Could you check a few things on this model? Use its own coordinates, in mm. Coordinates: 2 decimals unless noted, no trailing zeros. Write each loop counter-clockwise with the first axis right and the second up, starting at its lowest first coordinate (ties: lowest second). Pieces come first, ordered by that corner, then holes. Notation, with made-up numbers: M 54,48.5 L 92,48.5 A10 ccw 92,63.5 Z; hole C -14,46 d6. An arc over 180 degrees is marked long. Write item = value, one per line.
```python
from build123d import *

# Parameters (mm, degrees)
BOSS_EXTRUDE1_DEPTH = 6
SKETCH2_R           = 2.25
CUT_EXTRUDE1_DEPTH  = 20


with BuildPart() as part:
    # Sketch1 → Boss-Extrude1 (new, symmetric)
    with BuildSketch(Plane(origin=(0, 0, 0), x_dir=(0, 0, -1), z_dir=(1, 0, 0))):
        with BuildLine():
            Line((-1, 7.433034374), (-1, 15))
            Line((-1, 15), (-11, 15))
            Line((-11, 15), (-11, -15))
            Line((-11, -15), (-1, -15))
            Line((-1, -15), (-1, -7.433034374))
            ThreePointArc((-1, -7.433034374), (-7.5, 0), (-1, 7.433034374))
        make_face()
    extrude(amount=BOSS_EXTRUDE1_DEPTH, both=True)

    # Sketch2 → Cut-Extrude1 (cut, through all)
    with BuildSketch(Plane.XY.offset(11)):
        with Locations((0, 11)):
            Circle(SKETCH2_R)
        with Locations((0, -11)):
            Circle(SKETCH2_R)
    extrude(amount=-CUT_EXTRUDE1_DEPTH, mode=Mode.SUBTRACT)


solid = part.part
```
Item 1: Imagine slicing it at A-A (y = -11). Write out the boundary of the cut face in (x, z).
Numbers:
outline = M -6,1 L -2.25,1 L -2.25,11 L -6,11 Z; M 2.25,1 L 6,1 L 6,11 L 2.25,11 Z
Item 2: If we mould it in two halves opening along Y, with no side actions, what happens to faces 1 (the face through (-0.29, -8.77, 6.07)), 2 (the face through (0, -15, 6)), 3 (the face through (1.4, -13, 1))? For each: pulls with the +Y half, pulls with the -Y half, needs draft (parallel to the pull), parting line crosses it, or undercut.
Numbers:
face_1 = undercut
face_2 = pulls with the -Y half
face_3 = needs draft
Item 3: If I drill on line 1 along Y through (x, z) = (0, 8); line 2 along Y through (x, z) = (0.25, 5.75); line 3 along Y through (x, z) = (-1.5, 8.5), over which ranges is the centre line in solid material (lowest first)?
Numbers:
line_1 = -15 to -13.25, -8.75 to 8.75, 13.25 to 15
line_2 = -15 to -13.24, -8.76 to -4.82, 4.82 to 8.76, 13.24 to 15
line_3 = -15 to -12.68, -9.32 to 9.32, 12.68 to 15
Item 4: I'm going to push flat-ended pins straight in: P1, Ø1.5, axis at x = 4, y = -2, coming from the -Z side; P2, Ø1.5, axis at x = 4, y = -0.5, coming from the -Z side. Where does each tip first touch, or does it pass through?
Numbers:
P1 = 6.98
P2 = 7.4
Item 5: Imagine slicing it at C-C (x = 0). Write out the boundary of the cut face in (y, z), and give its area (3 significant figures).
Numbers:
outline = M -15,1 L -13.25,1 L -13.25,11 L -15,11 Z; M -8.75,1 L -7.43,1 A7.5 cw 7.43,1 L 8.75,1 L 8.75,11 L -8.75,11 Z; M 13.25,1 L 15,1 L 15,11 L 13.25,11 Z
area = 137 mm²
Item 6: Imagine slicing it at D-D (z = 9). Write out the boundary of the cut face in (x, y), and give its area (3 significant figures).
Numbers:
outline = M -6,-15 L 6,-15 L 6,15 L -6,15 Z; hole C 0,-11 d4.5; hole C 0,11 d4.5
area = 328 mm²
Item 7: Imagine slicing it at B-B (z = 4.25). Write out the boundary of the cut face in (x, y).
Numbers:
outline = M -6,-15 L 6,-15 L 6,-6.18 L -6,-6.18 Z; M -6,6.18 L 6,6.18 L 6,15 L -6,15 Z; hole C 0,-11 d4.5; hole C 0,11 d4.5
